Work out the finished part from the listing and answer in its coordinate system (mm). Round coordinates to 2 decimals unless told otherwise and drop trailing zeros. Order: outer loops, then holes, each group sorted by start corner. A loop starts at its lowest first (then second) coordinate and runs counter-clockwise, first axis right, second up. Notation, with made-up numbers: (42, 85.5) - (46, 85.5) arc R16 cw to (46, 91.5) - close; hole circle Ø2 at (-37.75, -31). An arc over 180 degrees is marked (long way). One line per question, with ' | ' between items. Start each with the question number.
from build123d import *

# Parameters (mm, degrees)
ESBO_O1_W                         = 130
ESBO_O1_H                         = 55.25
RESSALTO_EXTRUS_O1_DEPTH          = 2.5
ESBO_O2_W                         = 130
ESBO_O2_H                         = 55.25
ESBO_O2_W_2                       = 125
ESBO_O2_H_2                       = 52.75
CORTE_EXTRUS_O1_DEPTH             = 1.25
FUROS_GUIA_COM_3_0MM2_D           = 3
FUROS_GUIA_COM_3_0MM2_CSINK_D     = 3.05
FUROS_GUIA_COM_3_0MM2_CSINK_ANGLE = 90


with BuildPart() as part:
    # Esboço1 → Ressalto-extrusão1 (new body)
    with BuildSketch(Plane.XY):
        with Locations((1.708397535, 5.726309707)):
            Rectangle(ESBO_O1_W, ESBO_O1_H)
    extrude(amount=RESSALTO_EXTRUS_O1_DEPTH)

    # Esboço2 → Corte-extrusão1 (cut)
    with BuildSketch(Plane.XY.offset(2.5)):
        with Locations((1.708397535, 5.726309707)):
            Rectangle(ESBO_O2_W, ESBO_O2_H)
        with Locations((1.708397535, 5.726309707)):
            Rectangle(ESBO_O2_W_2, ESBO_O2_H_2, mode=Mode.SUBTRACT)
    extrude(amount=-CORTE_EXTRUS_O1_DEPTH, mode=Mode.SUBTRACT)

    # Furos-guia com Ø3.0mm2 (through all)
    with Locations(Plane.XY.offset(2.5)):
        with Locations((-48.791602465, 22.551309707), (-48.791602465, -11.098690293), (52.208397535, -11.098690293), (52.208397535, 22.551309707)):
            CounterSinkHole(FUROS_GUIA_COM_3_0MM2_D / 2, FUROS_GUIA_COM_3_0MM2_CSINK_D / 2, counter_sink_angle=FUROS_GUIA_COM_3_0MM2_CSINK_ANGLE)


solid = part.part
1) Straight lines are drawn through the part: line 1 (X direction, y = -12, z = 0.2); line 2 (Y direction, x = -57, z = 1.7); line 3 (X direction, y = 6.5, z = 1.3). For each, find the intervals that lie inside material, in ascending order.
2) Determine the mould class of faces 1 (the flat face through (-18, -21, 1.25)), 2 (the cylindrical face through (-47.6, 21.64, 1.22)), 3 (the cylindrical face through (-47.6, -12.01, 1.22)) for opening direction X: released by +X, released by -X, zero draft, split by the parting line, or undercut.
3) Section C-C on z = 2.05 is taken. Give the vertices of the cut face in (x, y).
4) Section B-B on y = -6 is taken. Give the vertices of the cut face in (x, z).
5) Section A-A on x = 0.5 is taken. Give the vertices of the cut face in (y, z), and give its area (3 significant figures).
6) Flat-ended cylindrical pins translate along their axes: pin 1 (0.6 mm diameter, centred on y = 5.5, z = 2, fed in from -X); pin 2 (2.5 mm diameter, centred on x = -48.79, y = 22.55, fed in from +Z); pin 3 (1.4 mm diameter, centred on x = 22, z = 2, fed in from +Y); pin 4 (1 mm diameter, centred on x = 15.5, z = 2, fed in from -Y). Find the tip coordinate at first contact, or state that the pin passes through.
Recorded:
1) line 1: x = -63.29 to -49.99, -47.59 to 51.01, 53.41 to 66.71 | line 2: y = -20.65 to 32.1 | line 3: x = -60.79 to 64.21
2) face 1: zero draft | face 2: undercut | face 3: undercut
3) outline: (-60.79, -20.65) - (64.21, -20.65) - (64.21, 32.1) - (-60.79, 32.1) - close; hole circle Ø3 at (-48.79, -11.1); hole circle Ø3 at (-48.79, 22.55); hole circle Ø3 at (52.21, -11.1); hole circle Ø3 at (52.21, 22.55)
4) outline: (-63.29, 0) - (66.71, 0) - (66.71, 1.25) - (64.21, 1.25) - (64.21, 2.5) - (-60.79, 2.5) - (-60.79, 1.25) - (-63.29, 1.25) - close
5) outline: (-21.9, 0) - (33.35, 0) - (33.35, 1.25) - (32.1, 1.25) - (32.1, 2.5) - (-20.65, 2.5) - (-20.65, 1.25) - (-21.9, 1.25) - close | area: 135 mm²
6) pin 1: stops at x = -60.79 | pin 2: passes through | pin 3: stops at y = 32.1 | pin 4: stops at y = -20.65
